```python
from build123d import *

# Parameters (mm, degrees)
SKETCH1_W            = 343
SKETCH1_H            = 199.5
BOSS_EXTRUDE1_DEPTH  = 1
M6_CLEARANCE_HOLE1_D = 7


with BuildPart() as part:
    # Sketch1 → Boss-Extrude1 (new body)
    with BuildSketch(Plane(origin=(0, 0, 0), x_dir=(1, 0, 0), z_dir=(0, 1, 0))):
        with Locations((11.41106981, 0.534905995)):
            Rectangle(SKETCH1_W, SKETCH1_H)
        with BuildLine():
            Line((-7.985757833, -4.648175221), (8.711031725, 4.759089682))
            add(Edge.make_bspline(
                [(8.711031725, 4.759089682), (9.311815171, 5.097749627), (9.310461275, 5.963705422), (8.708323934, 6.300339691)],
                knots=[5, 5, 5, 5, 6, 6, 6, 6], degree=3))
            Line((8.708323934, 6.300339691), (-4.290635533, 13.569700018))
            add(Edge.make_bspline(
                [(-4.290635533, 13.569700018), (-4.841299002, 13.877540751), (-5.535211865, 13.729542386), (-5.914514518, 13.224942375)],
                knots=[0, 0, 0, 0, 1, 1, 1, 1], degree=3))
            add(Edge.make_bspline(
                [(-5.914514518, 13.224942375), (-8.626837761, 9.614826119), (-10.237508511, 5.130289637), (-10.237508511, 0.267137786)],
                knots=[1, 1, 1, 1, 2, 2, 2, 2], degree=3))
            add(Edge.make_bspline(
                [(-10.237508511, 0.267137786), (-10.237508511, -1.12306501), (-10.095266787, -2.478045848), (-9.837887089, -3.792378812)],
                knots=[2, 2, 2, 2, 3, 3, 3, 3], degree=3))
            add(Edge.make_bspline(
                [(-9.837887089, -3.792378812), (-9.673300918, -4.634295207), (-8.732839522, -5.069133419), (-7.985757833, -4.648175221)],
                knots=[3, 3, 3, 3, 4, 4, 4, 4], degree=3))
        make_face(mode=Mode.SUBTRACT)
        with BuildLine():
            Line((17.789899426, -0.591423265), (30.86115737, 6.677229102))
            add(Edge.make_bspline(
                [(30.86115737, 6.677229102), (31.413846515, 6.984728777), (31.653279344, 7.656292027), (31.419262097, 8.244213464)],
                knots=[1, 1, 1, 1, 2, 2, 2, 2], degree=3))
            add(Edge.make_bspline(
                [(31.419262097, 8.244213464), (29.075058949, 14.133504536), (24.219017634, 18.737245846), (18.168855853, 20.745837898)],
                knots=[2, 2, 2, 2, 3, 3, 3, 3], degree=3))
            add(Edge.make_bspline(
                [(18.168855853, 20.745837898), (17.350994359, 21.017443836), (16.504344496, 20.419714407), (16.502990601, 19.558161356)],
                knots=[3, 3, 3, 3, 4, 4, 4, 4], degree=3))
            Line((16.502990601, 19.558161356), (16.476574133, 0.182074892))
            add(Edge.make_bspline(
                [(16.476574133, 0.182074892), (16.475897185, -0.492537207), (17.200288203, -0.919252045), (17.789899426, -0.591423265)],
                knots=[5, 5, 5, 5, 6, 6, 6, 6], degree=3))
        make_face(mode=Mode.SUBTRACT)
        with BuildLine():
            Line((14.008386181, -5.768334993), (27.011157828, -13.039827191))
            add(Edge.make_bspline(
                [(27.011157828, -13.039827191), (27.561480239, -13.347667924), (28.25539827, -13.199679894), (28.634354697, -12.695410606)],
                knots=[1, 1, 1, 1, 2, 2, 2, 2], degree=3))
            add(Edge.make_bspline(
                [(28.634354697, -12.695410606), (31.349401234, -9.084963628), (32.961756602, -4.598391135), (32.961756602, 0.267137786)],
                knots=[2, 2, 2, 2, 3, 3, 3, 3], degree=3))
            add(Edge.make_bspline(
                [(32.961756602, 0.267137786), (32.961756602, 1.665463955), (32.818160982, 3.02822711), (32.558068326, 4.350022002)],
                knots=[3, 3, 3, 3, 4, 4, 4, 4], degree=3))
            add(Edge.make_bspline(
                [(32.558068326, 4.350022002), (32.392469317, 5.191587005), (31.451666864, 5.626094494), (30.704585174, 5.204123458)],
                knots=[4, 4, 4, 4, 5, 5, 5, 5], degree=3))
            Line((30.704585174, 5.204123458), (14.004996275, -4.227436377))
            add(Edge.make_bspline(
                [(14.004996275, -4.227436377), (13.404889777, -4.56643738), (13.40658473, -5.431711059), (14.008386181, -5.768334993)],
                knots=[6, 6, 6, 6, 7, 7, 7, 7], degree=3))
        make_face(mode=Mode.SUBTRACT)
        with BuildLine():
            Line((15.306606753, 5.498905809), (15.306606753, 20.417885097))
            add(Edge.make_bspline(
                [(15.306606753, 20.417885097), (15.306606753, 21.047115854), (14.841962166, 21.580168344), (14.218829107, 21.665846168)],
                knots=[1, 1, 1, 1, 2, 2, 2, 2], degree=3))
            add(Edge.make_bspline(
                [(14.218829107, 21.665846168), (13.284129519, 21.794538601), (12.331813785, 21.867018527), (11.362233297, 21.867018527)],
                knots=[2, 2, 2, 2, 3, 3, 3, 3], degree=3))
            add(Edge.make_bspline(
                [(11.362233297, 21.867018527), (5.758087119, 21.867018527), (0.665320765, 19.719905379), (-3.170684195, 16.217149949)],
                knots=[3, 3, 3, 3, 4, 4, 4, 4], degree=3))
            add(Edge.make_bspline(
                [(-3.170684195, 16.217149949), (-3.804989477, 15.638044336), (-3.687474435, 14.607502371), (-2.938020844, 14.188580184)],
                knots=[4, 4, 4, 4, 5, 5, 5, 5], degree=3))
            Line((-2.938020844, 14.188580184), (13.991927564, 4.727433328))
            add(Edge.make_bspline(
                [(13.991927564, 4.727433328), (14.580856672, 4.398260987), (15.306606753, 4.823952653), (15.306606753, 5.498905809)],
                knots=[6, 6, 6, 6, 7, 7, 7, 7], degree=3))
        make_face(mode=Mode.SUBTRACT)
        with BuildLine():
            Line((7.357446123, -4.930131749), (7.357446123, -19.87689174))
            add(Edge.make_bspline(
                [(7.357446123, -19.87689174), (7.357787181, -20.505445549), (7.821408594, -21.037815923), (8.443869873, -21.124852811)],
                knots=[1, 1, 1, 1, 2, 2, 2, 2], degree=3))
            add(Edge.make_bspline(
                [(8.443869873, -21.124852811), (9.397870225, -21.257947988), (10.37084062, -21.332112532), (11.361763051, -21.332112532)],
                knots=[2, 2, 2, 2, 3, 3, 3, 3], degree=3))
            add(Edge.make_bspline(
                [(11.361763051, -21.332112532), (16.964214275, -21.332112532), (22.054608728, -19.186699506), (25.890267463, -15.686310809)],
                knots=[3, 3, 3, 3, 4, 4, 4, 4], degree=3))
            add(Edge.make_bspline(
                [(25.890267463, -15.686310809), (26.52458308, -15.107541086), (26.407403928, -14.076663231), (25.657955505, -13.657405154)],
                knots=[4, 4, 4, 4, 5, 5, 5, 5], degree=3))
            Line((25.657955505, -13.657405154), (8.672461202, -4.158669603))
            add(Edge.make_bspline(
                [(8.672461202, -4.158669603), (8.083532094, -3.829486928), (7.357446123, -4.255188928), (7.357446123, -4.930131749)],
                knots=[6, 6, 6, 6, 7, 7, 7, 7], degree=3))
        make_face(mode=Mode.SUBTRACT)
        with BuildLine():
            Line((4.847907511, 1.148952756), (-8.149526948, -6.119709946))
            add(Edge.make_bspline(
                [(-8.149526948, -6.119709946), (-8.700185249, -6.427891736), (-8.938264182, -7.097418975), (-8.705605999, -7.683976181)],
                knots=[1, 1, 1, 1, 2, 2, 2, 2], degree=3))
            add(Edge.make_bspline(
                [(-8.705605999, -7.683976181), (-6.373928969, -13.563789984), (-1.538542313, -18.16516456), (4.489941634, -20.188659799)],
                knots=[2, 2, 2, 2, 3, 3, 3, 3], degree=3))
            add(Edge.make_bspline(
                [(4.489941634, -20.188659799), (5.308821133, -20.463650476), (6.158855735, -19.864220926), (6.158855735, -19.000637033)],
                knots=[3, 3, 3, 3, 4, 4, 4, 4], degree=3))
            Line((6.158855735, -19.000637033), (6.16292259, 0.377480275))
            add(Edge.make_bspline(
                [(6.16292259, 0.377480275), (6.16325848, 1.052433432), (5.437172508, 1.478466155), (4.847907511, 1.148952756)],
                knots=[5, 5, 5, 5, 6, 6, 6, 6], degree=3))
        make_face(mode=Mode.SUBTRACT)
    extrude(amount=BOSS_EXTRUDE1_DEPTH)

    # M6 Clearance Hole1 (through all)
    with Locations(Plane(origin=(-135.08893019, 1, -85.284905995), x_dir=(0, 0, 1), z_dir=(0, 1, 0))):
        with Locations((0, 0), (0.999444907, 29.983347209), (0.999444907, 263.016652791), (0, 293)):
            Hole(M6_CLEARANCE_HOLE1_D / 2)


solid = part.part
```
Design review of the part built by this model. Coordinates are the model's own, in mm. A direction names the side the tool comes from. Coordinates: 2 decimals unless noted, no trailing zeros. One line per question, with ' | ' between items.
Q1. To check wall thickness, follow line 1 along X through (y, z) = (0.5, 4.5); line 2 along Z through (x, y) = (-134.5, 0.25) (3 decimals). State the ranges of each line that lie inside material, in increasing order.
Answer key:
line 1: x = -160.09 to -9.43, -7.72 to -5.25, 6.16 to 7.47, 9.28 to 13.71, 32.43 to 182.91 | line 2: z = -100.285 to -88.735, -81.835 to 99.215
Q2. For faces 1 (the flat face through (9, 0, -2)), 2 (the flat face through (22.472, 0.493, -0.554)), list the 3-axis set-ups (+Z, -Z, +X, -X, +Y, -Y) from which the entire face can be reached by the end or side of a thin tool; tool diameter is ignored.
Answer key:
face 1: +Z, -Z, +X, -X, -Y | face 2: +Y, -Y
Q3. Consider section A-A, the plane y = 0.45. Give the number of separate pieces and of enclosed holes in the cut face, then the cut area to 3 significant figures.
Answer key:
separate pieces: 1 | enclosed holes: 10 | area: 67,000 mm2
